from build123d import *

# Parameters (mm, degrees)
F0_W     = 160
F0_H     = 75
F0_R     = 10.25
F1_DEPTH = 6
F2_W     = 160
F2_H     = 63.5
F3_DEPTH = 6
F4_R     = 10
F5_R     = 2.1
F6_DEPTH = 25


with BuildPart() as f1:
    # F0 (on Top) → F1 (new body)
    with BuildSketch(Plane.XY):
        Rectangle(F0_W, F0_H)
        with Locations((-59, 0)):
            Circle(F0_R, mode=Mode.SUBTRACT)
        Circle(F0_R, mode=Mode.SUBTRACT)
        with Locations((59, 0)):
            Circle(F0_R, mode=Mode.SUBTRACT)
    extrude(amount=F1_DEPTH)

    # F2 (on face) → F3 (join)
    with BuildSketch(Plane(origin=(0, 37.5, 0), x_dir=(-1, 0, 0), z_dir=(0, 1, 0))):
        with Locations((0, -31.75)):
            Rectangle(F2_W, F2_H)
    extrude(amount=-F3_DEPTH)

    # F4
    f4_edges = [f1.edges().sort_by_distance(p)[0] for p in [
        (0, 37.5, 6),
        (-80, 34.5, -63.5),
        (80, 34.5, -63.5),
        (80, -37.5, 3),
        (-80, -37.5, 3),
    ]]
    fillet(f4_edges, radius=F4_R)

    # F5 (on face) → F6 (cut)
    with BuildSketch(Plane.XZ.offset(-31.5)):
        with Locations((-60, -25.4)):
            Circle(F5_R)
        with Locations((-40, -25.4)):
            Circle(F5_R)
        with Locations((-20, -25.4)):
            Circle(F5_R)
        with Locations((0, -25.4)):
            Circle(F5_R)
        with Locations((20, -25.4)):
            Circle(F5_R)
        with Locations((40, -25.4)):
            Circle(F5_R)
        with Locations((60, -25.4)):
            Circle(F5_R)
    extrude(amount=-F6_DEPTH, mode=Mode.SUBTRACT)


solid = f1.part
Design review of the part built by this model. Coordinates are the model's own, in mm. A direction names the side the tool comes from. Round coordinates to 2 decimals unless told otherwise and drop trailing zeros. Write each loop counter-clockwise with the first axis right and the second up, starting at its lowest first coordinate (ties: lowest second). Pieces come first, ordered by that corner, then holes. Notation, with made-up numbers: (9.25, 79.5) - (19.25, 79.5) arc R22 ccw to (19.25, 89.5) - close; hole circle Ø1 at (63, -24). An arc over 180 degrees is marked (long way). Use a Markdown table: item, result. Add a question column.
1. For faces 1 (the face through (-1, -18, 0)), 2 (the face through (-2.222, -10.006, 2.958)), list the 3-axis set-ups (+Z, -Z, +X, -X, +Y, -Y) from which the entire face can be reached by the end or side of a thin tool; tool diameter is ignored.
2. We need section B-B (z = -25.4). Count the separate pieces of the cut face and the enclosed holes in it, then the cut area to 3 significant figures.
3. Wall thickness on probe 1 along Z at (x, y) = (45.5, 0.5); probe 2 along Y at (x, z) = (-22.5, -10.5); probe 3 along Y at (x, z) = (59, 4.6): over which ranges is each line inside the solid? List them lowest first.
4. Mouldability with a two-part tool opening along Y and no side actions: class faces 3 (the face through (1, 37.5, -33)), 4 (the face through (-49.223, 3.079, 2.958)), 5 (the face through (68.777, 3.079, 2.958)), 6 (the face through (-1, -37.5, 3)) as +Y half, -Y half, draft (parallel to the pull), parting line (faces both ways), or undercut.
5. We need section D-D (x = 33). State the section outline as (y, z) points, then the cut area to 3 significant figures.
6. We need section A-A (x = -20). State the section outline as (y, z) points, then the cut area to 3 significant figures.
7. Clearance check with flat-ended pins moving along their axes: pin 1 (1.5 mm diameter, centred on x = -8.5, y = 29.5, fed in from +Z); pin 2 (19 mm diameter, centred on x = -5.5, z = -20.5, fed in from -Y). State where each tip first meets the part, or that it passes through.
8. We need section C-C (y = 33.5). State the section outline as (x, z) points, then the cut area to 3 significant figures.
Output:
| question | item | result |
|---|---|---|
| 1 | face 1 | -Z, +X, -X, -Y |
| 1 | face 2 | +Z, -Z |
| 2 | separate pieces | 8 |
| 2 | enclosed holes | 0 |
| 2 | area | 784 mm2 |
| 3 | probe 1 | z = 0 to 6 |
| 3 | probe 2 | y = 31.5 to 37.5 |
| 3 | probe 3 | y = -37.5 to -10.25, 10.25 to 32.6 |
| 4 | face 3 | +Y half |
| 4 | face 4 | undercut |
| 4 | face 5 | undercut |
| 4 | face 6 | -Y half |
| 5 | outline | (-37.5, 0) - (31.5, 0) - (31.5, -63.5) - (37.5, -63.5) - (37.5, -4) arc R10 ccw to (27.5, 6) - (-37.5, 6) - close |
| 5 | area | 810 mm2 |
| 6 | outline | (-37.5, 0) - (31.5, 0) - (31.5, -23.3) - (37.5, -23.3) - (37.5, -4) arc R10 ccw to (27.5, 6) - (-37.5, 6) - close; (31.5, -63.5) - (37.5, -63.5) - (37.5, -27.5) - (31.5, -27.5) - close |
| 6 | area | 784 mm2 |
| 7 | pin 1 | stops at z = 5.92 |
| 7 | pin 2 | stops at y = 31.5 |
| 8 | outline | (-80, -53.5) arc R10 ccw to (-70, -63.5) - (70, -63.5) arc R10 ccw to (80, -53.5) - (80, 4) - (-80, 4) - close; hole circle Ø4.2 at (-60, -25.4); hole circle Ø4.2 at (-40, -25.4); hole circle Ø4.2 at (-20, -25.4); hole circle Ø4.2 at (0, -25.4); hole circle Ø4.2 at (20, -25.4); hole circle Ø4.2 at (40, -25.4); hole circle Ø4.2 at (60, -25.4) |
| 8 | area | 10,700 mm2 |
